Geometry check sheet. Reference: the model listing, model coordinates, mm. A direction names the side the tool comes from. Round coordinates to 2 decimals unless told otherwise and drop trailing zeros. Order: outer loops, then holes, each group sorted by start corner. A loop starts at its lowest first (then second) coordinate and runs counter-clockwise, first axis right, second up.
```python
from build123d import *

# Parameters (mm, degrees)
SKETCH1_R               = 14.224
BOSS_EXTRUDE1_DEPTH     = 40.894
CUT_EXTRUDE1_START      = -11.43
CUT_EXTRUDE1_DEPTH      = 11.43
CUT_EXTRUDE2_DEPTH      = 11.43
CUT_EXTRUDE3_DEPTH      = 49.495378625
CUT_EXTRUDE3_DEPTH_BACK = 49.495378625
SKETCH4_R               = 3.175
SKETCH5_R               = 2.54
CUT_EXTRUDE4_DEPTH      = 36.67592549
BOSS_EXTRUDE2_REACH     = 50.495
BOSS_EXTRUDE3_DEPTH     = 1.27


with BuildPart() as part:
    # Sketch1 → Boss-Extrude1 (new body)
    with BuildSketch(Plane(origin=(0, 0, 0), x_dir=(1, 0, 0), z_dir=(0, 1, 0))):
        with Locations(Location((0, 0, 0), (0, 0, 270))):
            Circle(SKETCH1_R)
    extrude(amount=BOSS_EXTRUDE1_DEPTH)

    # Sketch2 → Cut-Extrude1 (cut)
    with BuildSketch(Plane(origin=(0, 40.894, 0), x_dir=(1, 0, 0), z_dir=(0, 1, 0)).offset(CUT_EXTRUDE1_START)):
        with BuildLine():
            Line((7.62, 12.010735864), (7.62, -12.010735864))
            ThreePointArc((7.62, -12.010735864), (0, -14.224), (-7.62, -12.010735864))
            Line((-7.62, -12.010735864), (-7.62, 12.010735864))
            ThreePointArc((-7.62, 12.010735864), (0, 14.224), (7.62, 12.010735864))
        make_face()
    extrude(amount=CUT_EXTRUDE1_DEPTH, mode=Mode.SUBTRACT)

    # Sketch3 → Cut-Extrude2 (cut)
    with BuildSketch(Plane.XZ):
        with BuildLine():
            Line((-7.62, 12.010735864), (-7.62, -12.010735864))
            ThreePointArc((-7.62, -12.010735864), (0, -14.224), (7.62, -12.010735864))
            Line((7.62, -12.010735864), (7.62, 12.010735864))
            ThreePointArc((7.62, 12.010735864), (0, 14.224), (-7.62, 12.010735864))
        make_face()
    extrude(amount=-CUT_EXTRUDE2_DEPTH, mode=Mode.SUBTRACT)

    # Sketch4 → Cut-Extrude3 (cut, two sides: drawn at the far end of the back side and taken through both)
    with BuildSketch(Plane(origin=(-7.62, 0, 0), x_dir=(0, 0, -1), z_dir=(1, 0, 0)).offset(-CUT_EXTRUDE3_DEPTH_BACK)):
        with Locations(Location((0, 35.814, 0), (0, 0, 270))):
            Circle(SKETCH4_R)
        with Locations(Location((0, 5.08, 0), (0, 0, 270))):
            Circle(SKETCH4_R)
        with BuildLine():
            Line((-3.881359545, 39.091414848), (-12.010735864, 29.464))
            Line((-12.010735864, 29.464), (-12.010735864, 40.894))
            Line((-12.010735864, 40.894), (0, 40.894))
            ThreePointArc((0, 40.894), (-2.139758464, 40.42136733), (-3.881359545, 39.091414848))
        make_face()
        with BuildLine():
            Line((-3.881359545, 1.802585152), (-12.010735864, 11.43))
            Line((-12.010735864, 11.43), (-12.010735864, 0))
            Line((-12.010735864, 0), (0, 0))
            ThreePointArc((0, 0), (-2.139758464, 0.47263267), (-3.881359545, 1.802585152))
        make_face()
    extrude(amount=CUT_EXTRUDE3_DEPTH + CUT_EXTRUDE3_DEPTH_BACK, mode=Mode.SUBTRACT)

    # Sketch5 → Cut-Extrude4 (cut, through all)
    with BuildSketch(Plane(origin=(0, 29.464, 0), x_dir=(1, 0, 0), z_dir=(0, 1, 0))):
        with Locations(Location((0, 0, 0), (0, 0, 270))):
            Circle(SKETCH5_R)
    extrude(amount=-CUT_EXTRUDE4_DEPTH, mode=Mode.SUBTRACT)

    # Boss-Extrude2: up to this face of the body (flat: up to its plane)
    boss_extrude2_end = Plane(part.part.faces().sort_by_distance((7.62, 29.730021804, 0))[0])
    # Sketch6 → Boss-Extrude2 (add, up to the picked face)
    with BuildSketch(Plane(origin=(-7.62, 0, 0), x_dir=(0, 0, -1), z_dir=(1, 0, 0)), mode=Mode.PRIVATE) as boss_extrude2_sk1:
        Polygon((2.54, 29.464), (12.010735864, 29.464), (12.010735864, 30.734), (6.930735864, 30.734), align=None)
    boss_extrude2_tool1 = split(extrude(boss_extrude2_sk1.sketch, amount=BOSS_EXTRUDE2_REACH, mode=Mode.PRIVATE), bisect_by=boss_extrude2_end, keep=Keep.BOTH, mode=Mode.PRIVATE)
    add(boss_extrude2_tool1.solids().sort_by(Axis((-7.62, 30.035129, -8.262642), (1, 0, 0)))[0])

    # Sketch7 → Boss-Extrude3 (add)
    with BuildSketch(Plane(origin=(0, 29.464, 0), x_dir=(1, 0, 0), z_dir=(0, 1, 0))):
        with BuildLine():
            Line((-7.62, 12.010735864), (7.62, 12.010735864))
            ThreePointArc((7.62, 12.010735864), (0, 14.224), (-7.62, 12.010735864))
        make_face()
    extrude(amount=BOSS_EXTRUDE3_DEPTH)


solid = part.part
```
(1) Sectioned sample at B-B, the plane x = 12.25. Record the cut outline in (y, z) (3 decimals).
Returned:
outline: (0, -7.229) - (40.894, -7.229) - (40.894, 0) arc R5.08 ccw to (39.091, 3.881) - (35.127, 7.229) - (5.767, 7.229) - (1.803, 3.881) arc R5.08 ccw to (0, 0) - close; hole circle Ø6.35 at (5.08, 0); hole circle Ø6.35 at (35.814, 0)
(2) Depth check by flat-ended pin: P1, Ø6, axis at x = -8.5, y = 9.5, coming from the +Z side; P2, Ø3.5, axis at x = -2, z = -11.5, coming from the +Y side; P3, Ø3.5, axis at y = 37, z = -3.5, coming from the +X side. Enter the tip coordinate at first touch or a pass-through.
Returned:
P1: stops at z = 12.8
P2: stops at y = 30.73
P3: stops at x = 14.06
(3) Sectioned sample at A-A, the plane y = 5.08. Record the cut outline in (x, z) (3 decimals).
Returned:
outline: (-13.865, -3.175) arc R14.224 ccw to (-7.62, -12.011) - (-7.62, -3.175) - close; (-13.865, 3.175) - (-7.62, 3.175) - (-7.62, 6.649) - (-12.574, 6.649) arc R14.224 ccw to start; (7.62, -12.011) arc R14.224 ccw to (13.865, -3.175) - (7.62, -3.175) - close; (7.62, 3.175) - (13.865, 3.175) arc R14.224 ccw to (12.574, 6.649) - (7.62, 6.649) - close
(4) Material ranges on line 1 (Y direction, x = 12.5, z = -1); line 2 (Y direction, x = -5.75, z = -1.75); line 3 (Y direction, x = 1, z = -11.5), recorded low to high.
Returned:
line 1: y = 0 to 2.07, 8.09 to 32.8, 38.83 to 40.89
line 2: y = 11.43 to 29.46
line 3: y = 11.43 to 30.73
(5) Draft check along Z on faces 4 (the cylindrical face through (-10.97, 0.46, 2.11)), 5 (the flat face through (0, 30.734, -11)), 6 (the cylindrical face through (-11, 32.8, -1)). Enter one of: released by +Z, released by -Z, zero draft, split by the parting line, or undercut.
Returned:
face 4: released by +Z
face 5: zero draft
face 6: undercut
(6) Sectioned sample at C-C, the plane y = 10. Record the cut outline in (x, z).
Returned:
outline: (-9.25, 10.8) arc R14.22 ccw to (-7.62, -12.01) - (-7.62, 10.8) - close; (7.62, -12.01) arc R14.22 ccw to (9.25, 10.8) - (7.62, 10.8) - close
(7) Sectioned sample at D-D, the plane x = 3.5. Record the cut outline in (y, z).
Returned:
outline: (11.43, -13.79) - (30.73, -13.79) - (30.73, -6.93) - (29.46, -2.54) - (29.46, 13.79) - (11.43, 13.79) - close
(8) Set-up check for faces 1 (the cylindrical face through (-10.968, 40.434, 2.112)), 2 (the flat face through (0, 29.464, 6)), 3 (the flat face through (0, 11.43, -3)): record each of +Z, -Z, +X, -X, +Y, -Y from which the full face is reachable in a straight line by a thin tool's end or side.
Returned:
face 1: +Z, +X, -X, +Y
face 2: +Z, +Y
face 3: +Z, -Z, -Y
